from build123d import *

# Parameters (mm, degrees)
BOSS_EXTRU_1_DEPTH      = 10
ENL_V_MAT_EXTRU_1_DEPTH = 20
ENL_V_MAT_EXTRU_2_DEPTH = 20
ESQUISSE5_R             = 1.6
ENL_V_MAT_EXTRU_3_DEPTH = 20
ESQUISSE6_R             = 1.6
ENL_V_MAT_EXTRU_4_DEPTH = 20
CHANFREIN1_SIZE         = 2
ENL_V_MAT_EXTRU_5_DEPTH = 2
ENL_V_MAT_EXTRU_6_DEPTH = 2


with BuildPart() as part:
    # Esquisse1 → Boss.-Extru.1 (new body)
    with BuildSketch(Plane.XY):
        with BuildLine():
            Line((-20, 87.749643874), (0, 87.749643874))
            Line((0, 87.749643874), (0, 77.459666924))
            Line((0, 77.459666924), (-20, 77.459666924))
            ThreePointArc((-20, 77.459666924), (-56.568542495, 56.568542495), (-77.459666924, 20))
            Line((-77.459666924, 20), (-77.459666924, 0))
            Line((-77.459666924, 0), (-87.749643874, 0))
            Line((-87.749643874, 0), (-87.749643874, 20))
            ThreePointArc((-87.749643874, 20), (-63.639610307, 63.639610307), (-20, 87.749643874))
        make_face()
    extrude(amount=BOSS_EXTRU_1_DEPTH)

    # Esquisse2 → Enlèv. mat.-Extru.1 (cut)
    with BuildSketch(Plane.XZ):
        Polygon((-84.459666924, 10), (-77.459666924, 10), (-77.459666924, 0), (-84.459666924, 0), (-81.459666924, 2.5), (-81.459666924, 7.5), align=None)
    extrude(amount=-ENL_V_MAT_EXTRU_1_DEPTH, mode=Mode.SUBTRACT)

    # Esquisse4 → Enlèv. mat.-Extru.2 (cut)
    with BuildSketch(Plane(origin=(0, 0, 0), x_dir=(0, 0, -1), z_dir=(1, 0, 0))):
        Polygon((0, 84.459666924), (0, 77.459666924), (-10, 77.459666924), (-10, 84.459666924), (-7.5, 81.459666924), (-2.5, 81.459666924), align=None)
    extrude(amount=-ENL_V_MAT_EXTRU_2_DEPTH, mode=Mode.SUBTRACT)

    # Esquisse5 → Enlèv. mat.-Extru.3 (cut)
    with BuildSketch(Plane(origin=(-81.459666924, 0, 0), x_dir=(0, 0, -1), z_dir=(1, 0, 0))):
        with Locations(Location((-5, 5, 0), (0, 0, 90))):
            Circle(ESQUISSE5_R)
        with Locations(Location((-5, 15, 0), (0, 0, 90))):
            Circle(ESQUISSE5_R)
    extrude(amount=-ENL_V_MAT_EXTRU_3_DEPTH, mode=Mode.SUBTRACT)

    # Esquisse6 → Enlèv. mat.-Extru.4 (cut)
    with BuildSketch(Plane.XZ.offset(-81.459666924)):
        with Locations(Location((-5, 5.05896145, 0), (0, 0, 270))):
            Circle(ESQUISSE6_R)
        with Locations(Location((-15, 5.05896145, 0), (0, 0, 270))):
            Circle(ESQUISSE6_R)
    extrude(amount=-ENL_V_MAT_EXTRU_4_DEPTH, mode=Mode.SUBTRACT)

    # Chanfrein1
    chanfrein1_edges = [part.edges().sort_by_distance(p)[0] for p in [
        (-82.959666924, 0, 8.75),
        (-81.459666924, 0, 5),
        (-82.959666924, 0, 1.25),
        (0, 82.959666924, 1.25),
        (0, 81.459666924, 5),
        (0, 82.959666924, 8.75),
    ]]
    chamfer(chanfrein1_edges, length=CHANFREIN1_SIZE)

    # Esquisse7 → Enlèv. mat.-Extru.5 (cut)
    with BuildSketch(Plane.ZY.offset(87.749643874)):
        Polygon((2.2, 6.616580754), (2.2, 3.383419246), (5, 1.766838493), (7.8, 3.383419246), (7.8, 6.616580754), (5, 8.233161507), align=None)
        Polygon((7.8, 16.616580754), (5, 18.233161507), (2.2, 16.616580754), (2.2, 13.383419246), (5, 11.766838493), (7.8, 13.383419246), align=None)
    extrude(amount=-ENL_V_MAT_EXTRU_5_DEPTH, mode=Mode.SUBTRACT)

    # Esquisse8 → Enlèv. mat.-Extru.6 (cut)
    with BuildSketch(Plane(origin=(0, 87.749643874, 0), x_dir=(1, 0, 0), z_dir=(0, 1, 0))):
        Polygon((-3.383419246, -2.25896145), (-6.616580754, -2.25896145), (-8.233161507, -5.05896145), (-6.616580754, -7.85896145), (-3.383419246, -7.85896145), (-1.766838493, -5.05896145), align=None)
        Polygon((-13.383419246, -2.25896145), (-16.616580754, -2.25896145), (-18.233161507, -5.05896145), (-16.616580754, -7.85896145), (-13.383419246, -7.85896145), (-11.766838493, -5.05896145), align=None)
    extrude(amount=-ENL_V_MAT_EXTRU_6_DEPTH, mode=Mode.SUBTRACT)


solid = part.part
Verification items for the finished model (mm, model axes). A direction names the side the tool comes from. Coordinates: 2 decimals unless noted, no trailing zeros. Write each loop counter-clockwise with the first axis right and the second up, starting at its lowest first coordinate (ties: lowest second). Pieces come first, ordered by that corner, then holes. Notation, with made-up numbers: (-10.75, 42) - (15.25, 42) arc R25 ccw to (15.25, 67) - close; hole circle Ø8 at (75, -2). An arc over 180 degrees is marked (long way). Answer as a JSON object with one key per item and string values.
(1) Cross-section at A-A on y = 15. Record the cut outline in (x, z), plus the area to 3 significant figures.
Report:
{"outline": "(-87.75, 0) - (-84.46, 0) - (-81.46, 2.5) - (-81.46, 3.4) - (-85.75, 3.4) - (-85.75, 2.2) - (-87.75, 2.2) - close; (-87.75, 7.8) - (-85.75, 7.8) - (-85.75, 6.6) - (-81.46, 6.6) - (-81.46, 7.5) - (-84.46, 10) - (-87.75, 10) - close", "area": "30.5 mm^2"}
(2) Cross-section at B-B on x = -5. Record the cut outline in (y, z), plus the area to 3 significant figures.
Report:
{"outline": "(81.46, 2.5) - (84.46, 0) - (87.75, 0) - (87.75, 2.26) - (85.75, 2.26) - (85.75, 3.46) - (81.46, 3.46) - close; (81.46, 6.66) - (85.75, 6.66) - (85.75, 7.86) - (87.75, 7.86) - (87.75, 10) - (84.46, 10) - (81.46, 7.5) - close", "area": "30.5 mm^2"}
(3) Mould release check, pull along Z, two halves, no side actions. Record for faces 6 (the flat face through (-84.48, 1.01, 8.73)), 7 (the flat face through (-86.764, 2.586, 3.58)), 8 (the flat face through (-20, 80, 5)): pulls with the +Z half, pulls with the -Z half, needs draft (parallel to the pull), parting line crosses it, or undercut.
Report:
{"face 6": "pulls with the +Z half", "face 7": "undercut", "face 8": "needs draft"}
(4) Cross-section at C-C on z = 1. Record the cut outline in (x, y).
Report:
{"outline": "(-87.75, 0) - (-86.38, 0) - (-83.26, 2) - (-83.26, 20) - (-77.46, 20) arc R80 cw to (-20, 77.46) - (-20, 83.26) - (-2, 83.26) - (0, 86.38) - (0, 87.75) - (-20, 87.75) arc R90 ccw to (-87.75, 20) - close"}
(5) Tool access check on faces 1 (the flat face through (-84.01, 1.01, 1.66)), 2 (the flat face through (-86.764, 12.564, 6.38)), 3 (the flat face through (-11, 81.46, 5)), 4 (the flat face through (0, 86, 5)), 5 (the flat face through (-7.436, 86.764, 6.439)). Record the directions out of +Z, -Z, +X, -X, +Y, -Y that give a thin tool (end or side, any length) a straight path to the whole face; none if there is none.
Report:
{"face 1": "-Z, +X, -Y", "face 2": "-X", "face 3": "+Z, -Z, +X, -Y", "face 4": "+Z, -Z, +X, +Y, -Y", "face 5": "+Y"}
(6) Cross-section at D-D on x = -54.5. Record the cut outline in (y, z).
Report:
{"outline": "(58.56, 0) - (71.62, 0) - (71.62, 10) - (58.56, 10) - close"}
(7) Thickness scan on line 1 along X through (y, z) = (83, 4.5); line 2 along Z through (x, y) = (-84, 15); line 3 along Z through (x, y) = (-83.75, 5). Record the ranges inside material, lowest first.
Report:
{"line 1": "-34.8 to -16.5, -13.5 to -6.5, -3.5 to -0.46", "line 2": "0.38 to 3.4, 6.6 to 9.62", "line 3": "0.59 to 3.4, 6.6 to 9.41"}
(8) Gauge pin test, flat ends, axial feed: pin 1 Ø5 at (y, z) = (61, 2.5) entering from +X; pin 2 Ø3 at (x, z) = (-76.5, 9) entering from +Y; pin 3 Ø1 at (x, z) = (-49.5, 4) entering from +Y. Record the tip position at first contact, or that the pin passes through.
Report:
{"pin 1": "x = -48.66", "pin 2": "y = 49.75", "pin 3": "y = 75.49"}
